Input: part model. Units: mm. Frame: model coordinates. Give positions to 0.01 mm unless a question says otherwise; leave off trailing zeros. Loops run counter-clockwise (first coordinate to the right, second up) from the corner with the lowest first, then second, coordinate; pieces in that order, holes last. Notation, with made-up numbers: (66.25, 6.5) -> (75.25, 6.5) arc R15 cw to (75.25, 27.5) -> close; hole circle Ø1 at (39, 37.25). An arc over 180 degrees is marked (long way). Use CSV: the item, a comma, the result in double quotes.
```python
from build123d import *

# Parameters (mm, degrees)
SKETCH1_W                                       = 100
SKETCH1_H                                       = 170
BOSS_EXTRUDE1_DEPTH                             = 3
M3_CLEARANCE_HOLE1_D                            = 3.4
M3_CLEARANCE_HOLE1_DEPTH                        = 7.5
M3_CLEARANCE_HOLE1_TIP                          = 1.021463052
FILLET1_R                                       = 5
CSK_FOR_M3_FLAT_HEAD_MACHINE_SCREW1_D           = 3.4
CSK_FOR_M3_FLAT_HEAD_MACHINE_SCREW1_DEPTH       = 7.5
CSK_FOR_M3_FLAT_HEAD_MACHINE_SCREW1_CSINK_D     = 6.3
CSK_FOR_M3_FLAT_HEAD_MACHINE_SCREW1_CSINK_ANGLE = 90
CSK_FOR_M3_FLAT_HEAD_MACHINE_SCREW1_TIP         = 1.021463052


with BuildPart() as part:
    # Sketch1 → Boss-Extrude1 (new body)
    with BuildSketch(Plane.XY):
        with Locations((50, 85)):
            Rectangle(SKETCH1_W, SKETCH1_H)
    extrude(amount=BOSS_EXTRUDE1_DEPTH)

    # M3 Clearance Hole1
    with Locations(Plane.XY.offset(3)):
        with Locations((5, 165), (95, 165), (95, 5), (5, 5)):
            Hole(M3_CLEARANCE_HOLE1_D / 2, depth=M3_CLEARANCE_HOLE1_DEPTH)
            with Locations((0, 0, -(M3_CLEARANCE_HOLE1_DEPTH + M3_CLEARANCE_HOLE1_TIP / 2))):  # 118° drill point
                Cone(0, M3_CLEARANCE_HOLE1_D / 2, M3_CLEARANCE_HOLE1_TIP, mode=Mode.SUBTRACT)

    # Fillet1
    fillet1_edges = [part.edges().sort_by_distance(p)[0] for p in [
        (0, 170, 1.5),
        (100, 170, 1.5),
        (100, 0, 1.5),
        (0, 0, 1.5),
    ]]
    fillet(fillet1_edges, radius=FILLET1_R)

    # CSK for M3 Flat Head Machine Screw1
    with Locations(Plane.XY.offset(3)):
        with Locations((50, 165), (50, 5), (95, 85), (5, 85)):
            CounterSinkHole(CSK_FOR_M3_FLAT_HEAD_MACHINE_SCREW1_D / 2, CSK_FOR_M3_FLAT_HEAD_MACHINE_SCREW1_CSINK_D / 2, depth=CSK_FOR_M3_FLAT_HEAD_MACHINE_SCREW1_DEPTH, counter_sink_angle=CSK_FOR_M3_FLAT_HEAD_MACHINE_SCREW1_CSINK_ANGLE)
            with Locations((0, 0, -(CSK_FOR_M3_FLAT_HEAD_MACHINE_SCREW1_DEPTH + CSK_FOR_M3_FLAT_HEAD_MACHINE_SCREW1_TIP / 2))):  # 118° drill point
                Cone(0, CSK_FOR_M3_FLAT_HEAD_MACHINE_SCREW1_D / 2, CSK_FOR_M3_FLAT_HEAD_MACHINE_SCREW1_TIP, mode=Mode.SUBTRACT)


solid = part.part
```
1) Ray query, line 1 (X direction, y = 85, z = 0.65); line 2 (Y direction, x = 95, z = 1.15); line 3 (Y direction, x = 50, z = 0.7). Return the intervals inside material, ascending.
From the geometry:
line 1,"x = 0 to 3.3, 6.7 to 93.3, 96.7 to 100"
line 2,"y = 0 to 3.3, 6.7 to 83.3, 86.7 to 163.3, 166.7 to 170"
line 3,"y = 0 to 3.3, 6.7 to 163.3, 166.7 to 170"
2) Contact query for flat-ended pins moving along their axis: pin 1 (4.5 mm diameter, centred on x = 5, y = 165, fed in from +Z); pin 2 (4 mm diameter, centred on x = 50, y = 165, fed in from +Z). Output: stop coordinate, or through.
From the geometry:
pin 1,"stops at z = 3"
pin 2,"stops at z = 1.85"
3) Mould query, pull axis X, two halves, no side actions, for faces 1 (the cylindrical face through (1, 168, 2)), 2 (the cylindrical face through (96.35, 163.97, 1.48)), 3 (the cylindrical face through (96.7, 5.07, 1.48)), 4 (the flat face through (49, 170, 1)). Classes: pulls with the +X half, pulls with the -X half, needs draft (parallel to the pull), parting line crosses it, or undercut.
From the geometry:
face 1,"pulls with the -X half"
face 2,"undercut"
face 3,"undercut"
face 4,"needs draft"
4) Section query A-A (y = 85). Return loops of the section in (x, z).
From the geometry:
outline,"(0, 0) -> (3.3, 0) -> (3.3, 1.55) -> (1.85, 3) -> (0, 3) -> close; (6.7, 0) -> (93.3, 0) -> (93.3, 1.55) -> (91.85, 3) -> (8.15, 3) -> (6.7, 1.55) -> close; (96.7, 0) -> (100, 0) -> (100, 3) -> (98.15, 3) -> (96.7, 1.55) -> close"
